Answer from the drawing. Dimensions are ordinates in mm from the lowest x, y and z of the part. A direction names the side the tool comes from. Coordinates: 2 decimals unless noted, no trailing zeros. Order: outer loops, then holes, each group sorted by start corner. A loop starts at its lowest first (then second) coordinate and runs counter-clockwise, first axis right, second up. Notation, with made-up numbers: (-29, -22.5) -> (-7, -22.5) arc R31 ccw to (-7, 3.5) -> close; hole circle Ø11 at (73.5, 25). An arc over 180 degrees is marked (long way). Answer in a Markdown table with one row per item.
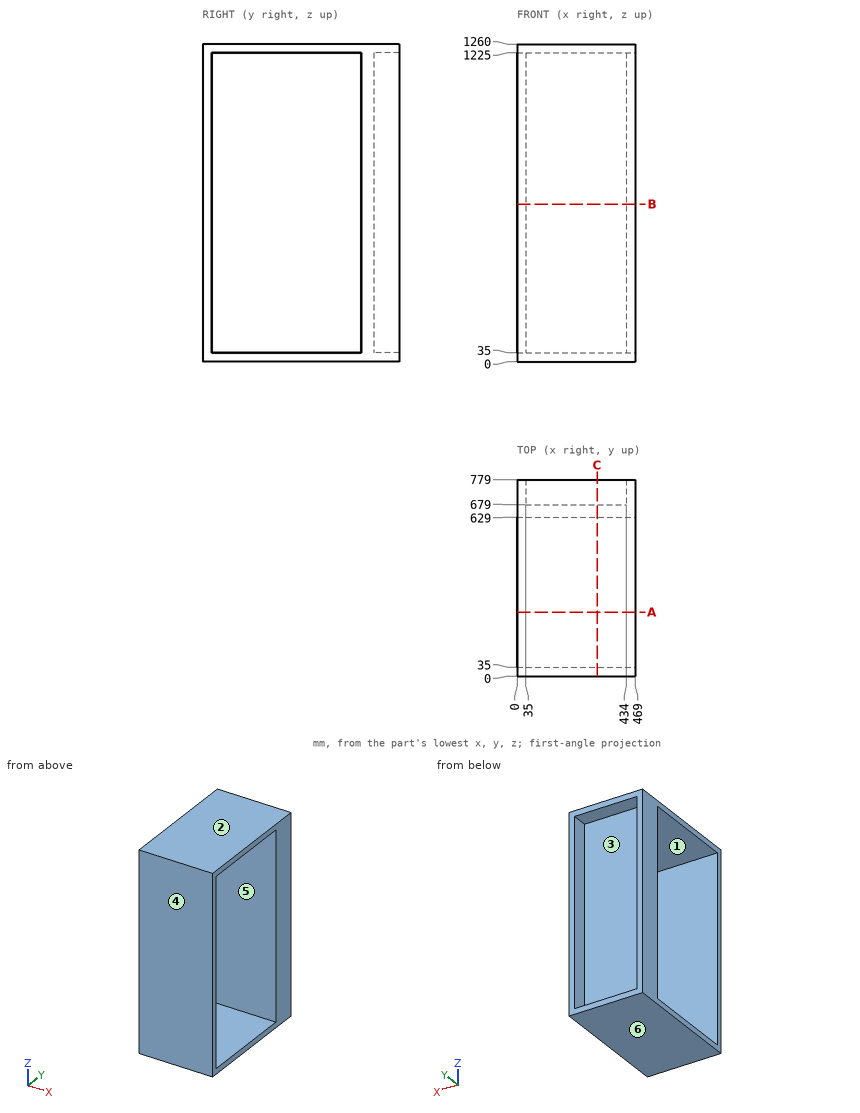
Q1. Given pin 1 (10 mm diameter, centred on x = 358, z = 938.5, fed in from +Y), flat-ended and moving along its own axis, determine where the tip first touches the part or whether it passes through.
Outcome:
| item | result |
|---|---|
| pin 1 | y = 679 |
Q2. For the marked faces 1, 2 and 3, determine the directions among +Z, -Z, +X, -X, +Y, -Y from which every point of the face is accessible in a straight line to the end or side of a thin tool.
Outcome:
| item | result |
|---|---|
| face 1 | +X, -X |
| face 2 | +Z, +X, -X, +Y, -Y |
| face 3 | +Y |
Q3. Consider line 1 (Z direction, x = 373, y = 450); line 2 (Y direction, x = 124.5, z = 769.5); line 3 (X direction, y = 706.5, z = 1000.5). Determine where each line is inside the solid, lowest interval first.
Outcome:
| item | result |
|---|---|
| line 1 | 0 to 35, 1225 to 1260 |
| line 2 | 0 to 35, 629 to 679 |
| line 3 | 0 to 35, 434 to 469 |
Q4. The part is cut by section B-B (z = 625). Write down the section's boundary in (x, y), then the cut area to 3 significant figures.
Outcome:
| item | result |
|---|---|
| outline | (0, 0) -> (469, 0) -> (469, 35) -> (0, 35) -> close; (0, 629) -> (469, 629) -> (469, 779) -> (434, 779) -> (434, 679) -> (35, 679) -> (35, 779) -> (0, 779) -> close |
| area | 46,900 mm² |
Q5. The part is cut by section C-C (x = 317.5). Write down the section's boundary in (y, z).
Outcome:
| item | result |
|---|---|
| outline | (0, 0) -> (779, 0) -> (779, 35) -> (679, 35) -> (679, 1225) -> (779, 1225) -> (779, 1260) -> (0, 1260) -> close; hole (35, 35) -> (629, 35) -> (629, 1225) -> (35, 1225) -> close |
Q6. For a pull along Y with two mould halves and no side action, classify the marked faces 4, 5 and 6 as pulls with the +Y half, pulls with the -Y half, needs draft (parallel to the pull), parting line crosses it, or undercut.
Outcome:
| item | result |
|---|---|
| face 4 | pulls with the -Y half |
| face 5 | undercut |
| face 6 | needs draft |
Q7. The part is cut by section A-A (y = 253). Write down the section's boundary in (x, z).
Outcome:
| item | result |
|---|---|
| outline | (0, 0) -> (469, 0) -> (469, 35) -> (0, 35) -> close; (0, 1225) -> (469, 1225) -> (469, 1260) -> (0, 1260) -> close |
